The model under review builds one solid part; all positions refer to its coordinate system, in mm. A direction names the side the tool comes from. Give positions to 0.01 mm unless a question says otherwise; leave off trailing zeros. Loops run counter-clockwise (first coordinate to the right, second up) from the corner with the lowest first, then second, coordinate; pieces in that order, holes last. Notation, with made-up numbers: M -12,89.25 L 36,89.25 A16 cw 36,109.25 Z; hole C 84.5,-5 d5. An arc over 180 degrees is marked long. Write item = value, one per line. Start each with the question number.
1. For faces 5 (the face through (-8.7, 0.5, 3.562)), 6 (the face through (0.03, 5.94, -1.75)), 7 (the face through (-13.75, 0.5, -4.7)), list the 3-axis set-ups (+Z, -Z, +X, -X, +Y, -Y) from which the entire face can be reached by the end or side of a thin tool; tool diameter is ignored.
2. For pin 1 (5 mm diameter, centred on x = 1.5, y = 8, fed in from +Z); pin 2 (0.9 mm diameter, centred on x = 13, z = -4.5, fed in from +Y); pin 3 (0.8 mm diameter, centred on x = 1, y = 0.5, fed in from +Z); pin 4 (1 mm diameter, centred on y = 8.5, z = -2.5, fed in from +X), all flat-tipped, find the tip position at first contact; note any pin that passes through.
3. We need section A-A on y = 7. Give the boundary of the cut face in (x, z).
4. Wall thickness on line 1 along Z through (x, y) = (-0.5, 3.5); line 2 along Y through (x, z) = (-5, 0); line 3 along X through (y, z) = (4, 2): over which ranges is each line inside the solid? List them lowest first. Write a range as from..to.
5. We need section C-C on x = 13. Give the boundary of the cut face in (y, z), then the cut area to 3 significant figures.
6. We need section B-B on y = 9. Give the boundary of the cut face in (x, z), then the cut area to 3 significant figures.
7. Draft analysis for pull direction Z (two halves, no side actions). For faces 1 (the face through (-5, 5, -0.5)), 2 (the face through (-7, 1, 4.5)), 3 (the face through (-4.875, 1.4, 2.9)), 4 (the face through (10, 1.5, 2)), state which applies: pulls with the +Z half, pulls with the -Z half, needs draft (parallel to the pull), parting line crosses it, or undercut.
from build123d import *

# Parameters (mm, degrees)
BOSS_EXTRUDE1_DEPTH     = 10
SKETCH2_W               = 18.5
SKETCH2_H               = 7.123903424
SKETCH2_R               = 1.05
BOSS_EXTRUDE2_DEPTH     = 1
SKETCH3_R               = 3.5
CUT_EXTRUDE1_DEPTH      = 8.5
BOSS_EXTRUDE3_DEPTH     = 4.5
SKETCH5_R               = 1.5
CUT_EXTRUDE2_DEPTH      = 4.5
M1_4X0_3_TAPPED_HOLE1_D = 1.1
SKETCH7_R               = 2.75
SKETCH7_R_2             = 1.75
BOSS_EXTRUDE4_DEPTH     = 1
SKETCH8_R               = 2
CUT_EXTRUDE3_DEPTH      = 1


with BuildPart() as part:
    # Sketch1 → Boss-Extrude1 (new body)
    with BuildSketch(Plane(origin=(0, 0, 0), x_dir=(1, 0, 0), z_dir=(0, 1, 0))):
        with BuildLine():
            ThreePointArc((10.063508327, -0.5), (10, 0), (10.063508327, 0.5))
            Line((10.063508327, 0.5), (7.527864045, 0.5))
            ThreePointArc((7.527864045, 0.5), (7.5, 0), (7.527864045, -0.5))
            Line((7.527864045, -0.5), (10.063508327, -0.5))
        make_face()
        with BuildLine():
            Line((7.527864045, 0.5), (10.063508327, 0.5))
            ThreePointArc((10.063508327, 0.5), (12.252008585, 1.984059393), (14, 0))
            ThreePointArc((14, 0), (12.252008585, -1.984059393), (10.063508327, -0.5))
            Line((10.063508327, -0.5), (7.527864045, -0.5))
            ThreePointArc((7.527864045, -0.5), (12.250387902, -4.493028589), (16.5, 0))
            ThreePointArc((16.5, 0), (12.250387902, 4.493028589), (7.527864045, 0.5))
        make_face()
        with BuildLine():
            ThreePointArc((-7.5, 0), (-7.506971411, 0.250387902), (-7.527864045, 0.5))
            Line((-7.527864045, 0.5), (-10.063508327, 0.5))
            ThreePointArc((-10.063508327, 0.5), (-10.015940607, 0.252008585), (-10, 0))
            ThreePointArc((-10, 0), (-10.015940607, -0.252008585), (-10.063508327, -0.5))
            Line((-10.063508327, -0.5), (-7.527864045, -0.5))
            ThreePointArc((-7.527864045, -0.5), (-7.506971411, -0.250387902), (-7.5, 0))
        make_face()
        with BuildLine():
            Line((-10.063508327, 0.5), (-7.527864045, 0.5))
            ThreePointArc((-7.527864045, 0.5), (-16.5, 0), (-7.527864045, -0.5))
            Line((-7.527864045, -0.5), (-10.063508327, -0.5))
            ThreePointArc((-10.063508327, -0.5), (-14, 0), (-10.063508327, 0.5))
        make_face()
        with BuildLine():
            ThreePointArc((7.527864045, -0.5), (7.5, 0), (7.527864045, 0.5))
            Line((7.527864045, 0.5), (1.677050983, 0.5))
            ThreePointArc((1.677050983, 0.5), (1.731666715, 0.252646769), (1.75, 0))
            ThreePointArc((1.75, 0), (1.731666715, -0.252646769), (1.677050983, -0.5))
            Line((1.677050983, -0.5), (7.527864045, -0.5))
        make_face()
        with BuildLine():
            ThreePointArc((-1.677050983, -0.5), (-1.75, 0), (-1.677050983, 0.5))
            Line((-1.677050983, 0.5), (-7.527864045, 0.5))
            ThreePointArc((-7.527864045, 0.5), (-7.506971411, 0.250387902), (-7.5, 0))
            ThreePointArc((-7.5, 0), (-7.506971411, -0.250387902), (-7.527864045, -0.5))
            Line((-7.527864045, -0.5), (-1.677050983, -0.5))
        make_face()
        with BuildLine():
            ThreePointArc((1.75, 0), (1.731666715, 0.252646769), (1.677050983, 0.5))
            Line((1.677050983, 0.5), (0.923309266, 0.5))
            ThreePointArc((0.923309266, 0.5), (1.017834645, 0.257900437), (1.05, 0))
            ThreePointArc((1.05, 0), (1.017834645, -0.257900437), (0.923309266, -0.5))
            Line((0.923309266, -0.5), (1.677050983, -0.5))
            ThreePointArc((1.677050983, -0.5), (1.731666715, -0.252646769), (1.75, 0))
        make_face()
        with BuildLine():
            Line((-0.923309266, 0.5), (-1.677050983, 0.5))
            ThreePointArc((-1.677050983, 0.5), (-1.75, 0), (-1.677050983, -0.5))
            Line((-1.677050983, -0.5), (-0.923309266, -0.5))
            ThreePointArc((-0.923309266, -0.5), (-1.05, 0), (-0.923309266, 0.5))
        make_face()
        with BuildLine():
            Line((0.923309266, 0.5), (1.677050983, 0.5))
            ThreePointArc((1.677050983, 0.5), (0, 1.75), (-1.677050983, 0.5))
            Line((-1.677050983, 0.5), (-0.923309266, 0.5))
            ThreePointArc((-0.923309266, 0.5), (0, 1.05), (0.923309266, 0.5))
        make_face()
        with BuildLine():
            ThreePointArc((-1.677050983, -0.5), (0, -1.75), (1.677050983, -0.5))
            Line((1.677050983, -0.5), (0.923309266, -0.5))
            ThreePointArc((0.923309266, -0.5), (0, -1.05), (-0.923309266, -0.5))
            Line((-0.923309266, -0.5), (-1.677050983, -0.5))
        make_face()
    extrude(amount=BOSS_EXTRUDE1_DEPTH)

    # Sketch2 → Boss-Extrude2 (add)
    # profile 1 of 5: a face of its own
    with BuildSketch(Plane(origin=(0, 0, 0), x_dir=(1, 0, 0), z_dir=(0, 1, 0))):
        with BuildLine():
            Line((-12.25, 5.25), (-13.75, 5.25))
            Line((-13.75, 5.25), (-13.75, 0.968245837))
            ThreePointArc((-13.75, 0.968245837), (-13.121649841, 1.655868846), (-12.25, 1.984313483))
            Line((-12.25, 1.984313483), (-12.25, 5.25))
        make_face()
    # profile 2 of 5: a face of its own
    with BuildSketch(Plane(origin=(0, 0, 0), x_dir=(1, 0, 0), z_dir=(0, 1, 0))):
        with BuildLine():
            ThreePointArc((-12.25, -1.984313483), (-13.121649841, -1.655868846), (-13.75, -0.968245837))
            Line((-13.75, -0.968245837), (-13.75, -5.25))
            Line((-13.75, -5.25), (-12.25, -5.25))
            Line((-12.25, -5.25), (-12.25, -1.984313483))
        make_face()
    # profile 3 of 5: a face of its own
    with BuildSketch(Plane(origin=(0, 0, 0), x_dir=(1, 0, 0), z_dir=(0, 1, 0))):
        with BuildLine():
            Line((13.75, 5.25), (12.25, 5.25))
            Line((12.25, 5.25), (12.25, 1.984313483))
            ThreePointArc((12.25, 1.984313483), (13.121649841, 1.655868846), (13.75, 0.968245837))
            Line((13.75, 0.968245837), (13.75, 5.25))
        make_face()
    # profile 4 of 5: a face of its own
    with BuildSketch(Plane(origin=(0, 0, 0), x_dir=(1, 0, 0), z_dir=(0, 1, 0))):
        with BuildLine():
            ThreePointArc((13.75, -0.968245837), (13.121649841, -1.655868846), (12.25, -1.984313483))
            Line((12.25, -1.984313483), (12.25, -5.25))
            Line((12.25, -5.25), (13.75, -5.25))
            Line((13.75, -5.25), (13.75, -0.968245837))
        make_face()
    # profile 5 of 5: a face of its own
    with BuildSketch(Plane(origin=(0, 0, 0), x_dir=(1, 0, 0), z_dir=(0, 1, 0))):
        Rectangle(SKETCH2_W, SKETCH2_H)
        with Locations(Location((0, 0, 0), (0, 0, 270))):
            Circle(SKETCH2_R, mode=Mode.SUBTRACT)
    extrude(amount=BOSS_EXTRUDE2_DEPTH)

    # Sketch3 → Cut-Extrude1 (cut)
    with BuildSketch(Plane(origin=(0, 10, 0), x_dir=(1, 0, 0), z_dir=(0, 1, 0))):
        with Locations(Location((-12, 0, 0), (0, 0, 270))):
            Circle(SKETCH3_R)
        with Locations(Location((12, 0, 0), (0, 0, 270))):
            Circle(SKETCH3_R)
    extrude(amount=-CUT_EXTRUDE1_DEPTH, mode=Mode.SUBTRACT)

    # Sketch4 → Boss-Extrude3 (add, symmetric)
    with BuildSketch(Plane.XY):
        with BuildLine():
            Line((-8.125, 0), (-4.875, 0))
            Line((-4.875, 0), (-4.875, 2))
            ThreePointArc((-4.875, 2), (-6.5, 3.625), (-8.125, 2))
            Line((-8.125, 2), (-8.125, 0))
        make_face()
        with BuildLine():
            Line((8.125, 0), (4.875, 0))
            Line((4.875, 0), (4.875, 2))
            ThreePointArc((4.875, 2), (6.5, 3.625), (8.125, 2))
            Line((8.125, 2), (8.125, 0))
        make_face()
    extrude(amount=BOSS_EXTRUDE3_DEPTH, both=True)

    # Sketch5 → Cut-Extrude2 (cut, symmetric)
    with BuildSketch(Plane.XY):
        with Locations((-5, 7)):
            Circle(SKETCH5_R)
        with Locations((5, 7)):
            Circle(SKETCH5_R)
    extrude(amount=CUT_EXTRUDE2_DEPTH, both=True, mode=Mode.SUBTRACT)

    # M1.4x0.3 Tapped Hole1 (through all)
    with Locations(Plane(origin=(-6.5, 2, 4.5), x_dir=(1, 0, 0), z_dir=(0, 0, 1))):
        with Locations((0, 0), (13, 0)):
            Hole(M1_4X0_3_TAPPED_HOLE1_D / 2)

    # Sketch7 → Boss-Extrude4 (add)
    with BuildSketch(Plane(origin=(0, 1, 0), x_dir=(1, 0, 0), z_dir=(0, 1, 0))):
        Circle(SKETCH7_R)
        Circle(SKETCH7_R_2, mode=Mode.SUBTRACT)
    extrude(amount=BOSS_EXTRUDE4_DEPTH)

    # Sketch8 → Cut-Extrude3 (cut)
    with BuildSketch(Plane.XZ):
        with Locations(Location((0, 0, 0), (0, 0, 270))):
            Circle(SKETCH8_R)
    extrude(amount=-CUT_EXTRUDE3_DEPTH, mode=Mode.SUBTRACT)


solid = part.part
Final values:
q1.face_5 = +Z, +Y, -Y
q1.face_6 = -Z, +Y
q1.face_7 = -Z, -X, +Y, -Y
q2.pin_1 = 1.75
q2.pin_2 = 10
q2.pin_3 = 3.56
q2.pin_4 = 16.03
q3.outline = M -7.53,-0.5 L -6.5,-0.5 L -6.5,0.5 L -7.53,0.5 A4.5 ccw long Z; M -3.5,-0.5 L -1.68,-0.5 A1.75 ccw 1.68,-0.5 L 3.5,-0.5 L 3.5,0.5 L 1.68,0.5 A1.75 ccw -1.68,0.5 L -3.5,0.5 Z; M 6.5,-0.5 L 7.53,-0.5 A4.5 ccw long 7.53,0.5 L 6.5,0.5 Z; hole C -12,0 d7; hole C 0,0 d2.1; hole C 12,0 d7
q4.line_1 = -1.68..-0.92, 0.92..1.68
q4.line_2 = 0..5.5, 8.5..10
q4.line_3 = -16.03..-14.87, -9.13..-7.97, 7.97..9.13, 14.87..16.03
q5.outline = M 0,-5.25 L 1,-5.25 L 1,-4.39 L 10,-4.39 L 10,-3.35 L 1.5,-3.35 L 1.5,-1.73 L 0,-1.73 Z; M 0,1.73 L 1.5,1.73 L 1.5,3.35 L 10,3.35 L 10,4.39 L 1,4.39 L 1,5.25 L 0,5.25 Z
q5.area = 27.3 mm²
q6.outline = M -7.53,-0.5 L -1.68,-0.5 A1.75 ccw 1.68,-0.5 L 7.53,-0.5 A4.5 ccw long 7.53,0.5 L 1.68,0.5 A1.75 ccw -1.68,0.5 L -7.53,0.5 A4.5 ccw long Z; hole C -12,0 d7; hole C 0,0 d2.1; hole C 12,0 d7
q6.area = 68.0 mm²
q7.face_1 = pulls with the -Z half
q7.face_2 = pulls with the +Z half
q7.face_3 = needs draft
q7.face_4 = undercut
